```python
from build123d import *

# Parameters (mm, degrees)
SKETCH1_W           = 62
SKETCH1_H           = 52
BOSS_EXTRUDE1_DEPTH = 2.778125
CUT_EXTRUDE1_DEPTH  = 10
SKETCH2_W           = 40
SKETCH2_H           = 10
CUT_EXTRUDE2_DEPTH  = 10
FILLET1_R           = 7
FILLET2_R           = 7
SKETCH4_R           = 2.1
SKETCH4_R_2         = 1.8
SKETCH4_R_3         = 12
CUT_EXTRUDE3_DEPTH  = 10


with BuildPart() as part:
    # Sketch1 → Boss-Extrude1 (new body)
    with BuildSketch(Plane.XY):
        with Locations((-31, 4.465517241)):
            Rectangle(SKETCH1_W, SKETCH1_H)
    extrude(amount=BOSS_EXTRUDE1_DEPTH)

    # Sketch3 → Cut-Extrude1 (cut)
    with BuildSketch(Plane.XY.offset(2.778125)):
        Polygon((-20, 30.465517241), (0, 21.802451622), (0, 30.465517241), align=None)
    extrude(amount=-CUT_EXTRUDE1_DEPTH, mode=Mode.SUBTRACT)

    # Sketch2 → Cut-Extrude2 (cut)
    with BuildSketch(Plane.XY.offset(2.778125)):
        with Locations((-42, -16.534482759)):
            Rectangle(SKETCH2_W, SKETCH2_H)
    extrude(amount=-CUT_EXTRUDE2_DEPTH, mode=Mode.SUBTRACT)

    # Fillet1
    fillet1_edges = [part.edges().sort_by_distance(p)[0] for p in [
        (-62, -11.534482759, 1.3890625),
        (-22, -21.534482759, 1.3890625),
        (-62, 30.465517241, 1.3890625),
        (0, -21.534482759, 1.3890625),
    ]]
    fillet(fillet1_edges, radius=FILLET1_R)

    # Fillet2
    fillet2_edges = [part.edges().sort_by_distance(p)[0] for p in [
        (0, 21.802451622, 1.3890625),
        (-20, 30.465517241, 1.3890625),
    ]]
    fillet(fillet2_edges, radius=FILLET2_R)

    # Sketch4 → Cut-Extrude3 (cut)
    with BuildSketch(Plane.XY.offset(2.778125)):
        with Locations((-10.925971148, -11.534482759)):
            Circle(SKETCH4_R)
        with Locations((-10.925971148, 14.465517241)):
            Circle(SKETCH4_R)
        with Locations((-56, -6.534482759)):
            Circle(SKETCH4_R_2)
        with Locations((-56, 24.465517241)):
            Circle(SKETCH4_R_2)
        with Locations((-25, 24.465517241)):
            Circle(SKETCH4_R_2)
        with Locations((-25, -6.534482759)):
            Circle(SKETCH4_R_2)
        with Locations((-41, 9.468169555)):
            Circle(SKETCH4_R_3)
    extrude(amount=-CUT_EXTRUDE3_DEPTH, mode=Mode.SUBTRACT)


solid = part.part
```
Model file for the job. Use its own axes, mm. A direction names the side the tool comes from. Give positions to 0.01 mm unless a question says otherwise; leave off trailing zeros. Loops run counter-clockwise (first coordinate to the right, second up) from the corner with the lowest first, then second, coordinate; pieces in that order, holes last. Notation, with made-up numbers: (84, 23) -> (134, 23) arc R34 ccw to (134, 62) -> close; hole circle Ø6 at (51.5, -6). An arc over 180 degrees is marked (long way). Write each question's results on one line, items separated by ' | '.
(1) Probe line 1 along Y through (x, z) = (-25, 1.95); line 2 along Y through (x, z) = (-12, 1.9); line 3 along X through (y, z) = (24.5, 2.65). List the from-to ranges inside material, lowest first.
Geometry results:
line 1: y = -11.53 to -8.33, -4.73 to 22.67, 26.27 to 30.47 | line 2: y = -21.53 to -13.34, -9.73 to 12.66, 16.27 to 27 | line 3: x = -61.92 to -57.8, -54.2 to -26.8, -23.2 to -6.23
(2) Cut at B-B on x = -41. List the corners of the cut face in (y, z).
Geometry results:
outline: (-11.53, 0) -> (-2.53, 0) -> (-2.53, 2.78) -> (-11.53, 2.78) -> close; (21.47, 0) -> (30.47, 0) -> (30.47, 2.78) -> (21.47, 2.78) -> close
(3) Cut at C-C on y = 1.5. List the corners of the cut face in (x, z).
Geometry results:
outline: (-62, 0) -> (-49.97, 0) -> (-49.97, 2.78) -> (-62, 2.78) -> close; (-32.03, 0) -> (0, 0) -> (0, 2.78) -> (-32.03, 2.78) -> close
(4) Flat gauge pins, fed straight in: pin 1 Ø6 at (x, y) = (-56, -6.53) entering from +Z; pin 2 Ø0.8 at (y, z) = (-13, 1) entering from -X; pin 3 Ø3.5 at (x, y) = (-10.93, 14.47) entering from +Z; pin 4 Ø1 at (x, z) = (-51.5, 0.5) entering from -Y. Where does each tip first touch, or does it go through?
Geometry results:
pin 1: stops at z = 2.78 | pin 2: stops at x = -22 | pin 3: passes through | pin 4: stops at y = -11.53
(5) Cut at D-D on z = 0.85. List the corners of the cut face in (x, y), and give its area (3 significant figures).
Geometry results:
outline: (-62, -4.53) arc R7 ccw to (-55, -11.53) -> (-22, -11.53) -> (-22, -14.53) arc R7 ccw to (-15, -21.53) -> (-7, -21.53) arc R7 ccw to (0, -14.53) -> (0, 17.21) arc R7 ccw to (-4.22, 23.63) -> (-18.67, 29.89) arc R7 ccw to (-21.45, 30.47) -> (-55, 30.47) arc R7 ccw to (-62, 23.47) -> close; hole circle Ø3.6 at (-56, -6.53); hole circle Ø3.6 at (-56, 24.47); hole circle Ø24 at (-41, 9.47); hole circle Ø3.6 at (-25, -6.53); hole circle Ø3.6 at (-25, 24.47); hole circle Ø4.2 at (-10.93, -11.53); hole circle Ø4.2 at (-10.93, 14.47) | area: 2,170 mm²
(6) Cut at A-A on x = -25. List the corners of the cut face in (y, z).
Geometry results:
outline: (-11.53, 0) -> (-8.33, 0) -> (-8.33, 2.78) -> (-11.53, 2.78) -> close; (-4.73, 0) -> (22.67, 0) -> (22.67, 2.78) -> (-4.73, 2.78) -> close; (26.27, 0) -> (30.47, 0) -> (30.47, 2.78) -> (26.27, 2.78) -> close
(7) Pull direction X, two halves, no side cores. Call faces 1 (the cylindrical face through (-25.23, 26.25, 1.41)), 2 (the flat face through (-39, -11.534, 1)), 3 (the cylindrical face through (-60.004, 28.361, 1.409)): released by +X, released by -X, zero draft, split by the parting line, or undercut.
Geometry results:
face 1: undercut | face 2: zero draft | face 3: released by -X
(8) Tool access for faces 4 (the cylindrical face through (-50.523, 2.166, 1.409)), 5 (the flat face through (-22, -13, 1)): list every direction of +Z, -Z, +X, -X, +Y, -Y with a clear straight run to the whole face (end or side of a thin tool).
Geometry results:
face 4: +Z, -Z | face 5: +Z, -Z, -X, -Y
